Part model, mm, in its own coordinate system. A direction names the side the tool comes from. Give positions to 0.01 mm unless a question says otherwise; leave off trailing zeros. Order: outer loops, then holes, each group sorted by start corner. A loop starts at its lowest first (then second) coordinate and runs counter-clockwise, first axis right, second up. Notation, with made-up numbers: M 19,-4.5 L 45,-4.5 A14 cw 45,3.5 Z; hole C -27,33.5 d7. An arc over 180 degrees is marked long. Answer as a JSON object with one key per item and string values.
from build123d import *

# Parameters (mm, degrees)
F1_DEPTH    = 8
F2_T1_DEPTH = 8


# Not quite as in the source:
# - a fillet or chamfer that OpenCascade refuses, or shapes differently, is made with other operations: its cross-section is extruded or revolved along the edge and cut away or added


with BuildPart() as f1:
    # F0 (on Top) → F1 (new body)
    with BuildSketch(Plane.XY):
        with BuildLine():
            ThreePointArc((12.9113873807, 7.6351866975), (14.4684278813, 3.9578522768), (15, 0))
            ThreePointArc((15, 0), (14.4684278813, -3.9578522768), (12.9113873807, -7.6351866975))
            Line((12.9113873807, -7.6351866975), (18.4852353, -7.6351866975))
            ThreePointArc((18.4852353, -7.6351866975), (19.6176541156, -3.8919978161), (20, 0))
            ThreePointArc((20, 0), (19.6176541156, 3.8919978161), (18.4852353, 7.6351866975))
            Line((18.4852353, 7.6351866975), (12.9113873807, 7.6351866975))
        make_face()
        with BuildLine():
            ThreePointArc((-12.9113873807, 7.6351866975), (0, 15), (12.9113873807, 7.6351866975))
            Line((12.9113873807, 7.6351866975), (18.4852353, 7.6351866975))
            ThreePointArc((18.4852353, 7.6351866975), (0, 20), (-18.4852353, 7.6351866975))
            Line((-18.4852353, 7.6351866975), (-12.9113873807, 7.6351866975))
        make_face()
        with BuildLine():
            Line((18.4852353, -7.6351866975), (12.9113873807, -7.6351866975))
            ThreePointArc((12.9113873807, -7.6351866975), (0, -15), (-12.9113873807, -7.6351866975))
            Line((-12.9113873807, -7.6351866975), (-18.4852353, -7.6351866975))
            ThreePointArc((-18.4852353, -7.6351866975), (0, -20), (18.4852353, -7.6351866975))
        make_face()
        with BuildLine():
            ThreePointArc((-12.9113873807, -7.6351866975), (-15, 0), (-12.9113873807, 7.6351866975))
            Line((-12.9113873807, 7.6351866975), (-18.4852353, 7.6351866975))
            ThreePointArc((-18.4852353, 7.6351866975), (-20, 0), (-18.4852353, -7.6351866975))
            Line((-18.4852353, -7.6351866975), (-12.9113873807, -7.6351866975))
        make_face()
        with BuildLine():
            Line((21.6526307541, 7.6351866975), (18.4852353, 7.6351866975))
            ThreePointArc((18.4852353, 7.6351866975), (19.6176541156, 3.8919978161), (20, 0))
            ThreePointArc((20, 0), (19.6176541156, -3.8919978161), (18.4852353, -7.6351866975))
            Line((18.4852353, -7.6351866975), (21.6526307541, -7.6351866975))
            ThreePointArc((21.6526307541, -7.6351866975), (20.1620412737, 0), (21.6526307541, 7.6351866975))
        make_face()
        with BuildLine():
            ThreePointArc((-18.4852353, -7.6351866975), (-20, 0), (-18.4852353, 7.6351866975))
            Line((-18.4852353, 7.6351866975), (-21.5730507637, 7.6351866975))
            ThreePointArc((-21.5730507637, 7.6351866975), (-20.4496870957, 3.8908164426), (-20.0704748243, 0))
            ThreePointArc((-20.0704748243, 0), (-20.4496870957, -3.8908164426), (-21.5730507637, -7.6351866975))
            Line((-21.5730507637, -7.6351866975), (-18.4852353, -7.6351866975))
        make_face()
        with BuildLine():
            Line((27.135123316, 7.6351866975), (21.6526307541, 7.6351866975))
            ThreePointArc((21.6526307541, 7.6351866975), (20.1620412737, 0), (21.6526307541, -7.6351866975))
            Line((21.6526307541, -7.6351866975), (27.135123316, -7.6351866975))
            Line((27.135123316, -7.6351866975), (27.135123316, -7.5155344287))
            ThreePointArc((27.135123316, -7.5155344287), (25.1620412737, 0), (27.135123316, 7.5155344287))
            Line((27.135123316, 7.5155344287), (27.135123316, 7.6351866975))
        make_face()
        with BuildLine():
            ThreePointArc((60.7620412737, 0), (44.3517049129, 19.9238680174), (21.6526307541, 7.6351866975))
            Line((21.6526307541, 7.6351866975), (27.135123316, 7.6351866975))
            Line((27.135123316, 7.6351866975), (27.135123316, 7.5155344287))
            ThreePointArc((27.135123316, 7.5155344287), (44.347151005, 14.7985108162), (55.7620412737, 0))
            ThreePointArc((55.7620412737, 0), (44.347151005, -14.7985108162), (27.135123316, -7.5155344287))
            Line((27.135123316, -7.5155344287), (27.135123316, -7.6351866975))
            Line((27.135123316, -7.6351866975), (21.6526307541, -7.6351866975))
            ThreePointArc((21.6526307541, -7.6351866975), (44.3517049129, -19.9238680174), (60.7620412737, 0))
        make_face()
        with BuildLine():
            Line((-27.135123316, 7.6351866975), (-21.5730507637, 7.6351866975))
            ThreePointArc((-21.5730507637, 7.6351866975), (-60.3704748243, 0), (-21.5730507637, -7.6351866975))
            Line((-21.5730507637, -7.6351866975), (-27.135123316, -7.6351866975))
            ThreePointArc((-27.135123316, -7.6351866975), (-55.3704748243, 0), (-27.135123316, 7.6351866975))
        make_face()
        with BuildLine():
            ThreePointArc((-20.0704748243, 0), (-20.4496870957, 3.8908164426), (-21.5730507637, 7.6351866975))
            Line((-21.5730507637, 7.6351866975), (-27.135123316, 7.6351866975))
            ThreePointArc((-27.135123316, 7.6351866975), (-25.5957427695, 3.9547076156), (-25.0704748243, 0))
            ThreePointArc((-25.0704748243, 0), (-25.5957427695, -3.9547076156), (-27.135123316, -7.6351866975))
            Line((-27.135123316, -7.6351866975), (-21.5730507637, -7.6351866975))
            ThreePointArc((-21.5730507637, -7.6351866975), (-20.4496870957, -3.8908164426), (-20.0704748243, 0))
        make_face()
    extrude(amount=F1_DEPTH)

    # F2: chamfer of 1 on 13 edges, made by hand

    # F2_s2 → F2_t1 (join)
    with BuildSketch(Plane.XY):
        with BuildLine():
            Line((20.9909460118, -7.6351866975), (21.9050819396, -8.2297788713))
            ThreePointArc((21.9050819396, -8.2297788713), (21.7829852925, -7.9487651651), (21.6526307541, -7.6351866975))
            Line((21.6526307541, -7.6351866975), (20.9909460118, -7.6351866975))
        make_face()
        with BuildLine():
            Line((-19.1424541452, -7.6351866975), (-18.2309087097, -8.2239873309))
            ThreePointArc((-18.2309087097, -8.2239873309), (-18.3538297184, -7.9458753243), (-18.4852353, -7.6351866975))
            Line((-18.4852353, -7.6351866975), (-19.1424541452, -7.6351866975))
        make_face()
        with BuildLine():
            Line((21.9050819396, 8.2297788713), (20.9909460118, 7.6351866975))
            Line((20.9909460118, 7.6351866975), (21.6526307541, 7.6351866975))
            ThreePointArc((21.6526307541, 7.6351866975), (21.7829852925, 7.9487651651), (21.9050819396, 8.2297788713))
        make_face()
        with BuildLine():
            Line((-18.2309087097, 8.2239873309), (-19.1424541452, 7.6351866975))
            Line((-19.1424541452, 7.6351866975), (-18.4852353, 7.6351866975))
            ThreePointArc((-18.4852353, 7.6351866975), (-18.3538297184, 7.9458753243), (-18.2309087097, 8.2239873309))
        make_face()
        with BuildLine():
            Line((19.1424541452, 7.6351866975), (18.2309087097, 8.2239873309))
            ThreePointArc((18.2309087097, 8.2239873309), (18.3538297184, 7.9458753243), (18.4852353, 7.6351866975))
            Line((18.4852353, 7.6351866975), (19.1424541452, 7.6351866975))
        make_face()
        with BuildLine():
            Line((19.1424541452, -7.6351866975), (18.2309087097, -8.2239873309))
            ThreePointArc((18.2309087097, -8.2239873309), (18.3538297184, -7.9458753243), (18.4852353, -7.6351866975))
            Line((18.4852353, -7.6351866975), (19.1424541452, -7.6351866975))
        make_face()
        with BuildLine():
            Line((-21.8264389289, -8.2269036385), (-20.9135835494, -7.6351866975))
            Line((-20.9135835494, -7.6351866975), (-21.5730507637, -7.6351866975))
            ThreePointArc((-21.5730507637, -7.6351866975), (-21.703929906, -7.9473306392), (-21.8264389289, -8.2269036385))
        make_face()
    extrude(amount=F2_T1_DEPTH)

    # F2_s3 → F2_t4 (revolve, cut)
    with BuildSketch(Plane(origin=(-10.2155381424, -17.5076147757, 0), x_dir=(0, 0, 1), z_dir=(0.5039727193, 0.8637195715, 0))):
        Polygon((8, -18.5892112809), (7, -19.5892112809), (8, -19.5892112809), align=None)
    revolve(axis=Axis((-40.2204748243, 0, 8), (0, 0, -1)), mode=Mode.SUBTRACT)

    # F2_s5 → F2_t6 (revolve, cut)
    with BuildSketch(Plane(origin=(0, 0, 0), x_dir=(0, 0, 1), z_dir=(0.5090124465, -0.8607591587, 0))):
        Polygon((7, 15), (8, 16), (8, 15), align=None)
    revolve(axis=Axis((0, 0, 8), (0, 0, -1)), mode=Mode.SUBTRACT)

    # F2_s7 → F2_t8 (revolve, cut)
    with BuildSketch(Plane(origin=(9.7630309126, 17.3122900606, 0), x_dir=(0, 0, 1), z_dir=(-0.4912114006, -0.8710403894, 0))):
        Polygon((8, -18.9440721866), (7, -19.9440721866), (8, -19.9440721866), align=None)
    revolve(axis=Axis((40.4620412737, 0, 8), (0, 0, -1)), mode=Mode.SUBTRACT)

    # F2_s9 → F2_t10 (revolve, cut)
    with BuildSketch(Plane(origin=(-10.2155381424, -17.5076147757, 0), x_dir=(0, 0, 1), z_dir=(0.5039727193, 0.8637195715, 0))):
        Polygon((0, -18.5892112809), (1, -19.5892112809), (0, -19.5892112809), align=None)
    revolve(axis=Axis((-40.2204748243, 0, 0), (0, 0, -1)), mode=Mode.SUBTRACT)

    # F2_s11 → F2_t12 (revolve, cut)
    with BuildSketch(Plane(origin=(0, 0, 0), x_dir=(0, 0, 1), z_dir=(0.5090124465, -0.8607591587, 0))):
        Polygon((1, 15), (0, 16), (0, 15), align=None)
    revolve(axis=Axis((0, 0, 0), (0, 0, -1)), mode=Mode.SUBTRACT)

    # F2_s13 → F2_t14 (revolve, cut)
    with BuildSketch(Plane(origin=(9.7630309126, 17.3122900606, 0), x_dir=(0, 0, 1), z_dir=(-0.4912114006, -0.8710403894, 0))):
        Polygon((0, -18.9440721866), (1, -19.9440721866), (0, -19.9440721866), align=None)
    revolve(axis=Axis((40.4620412737, 0, 0), (0, 0, -1)), mode=Mode.SUBTRACT)


solid = f1.part
1. Probe line 1 along Y through (x, z) = (40, 1.5); line 2 along X through (y, z) = (-7, 7.75); line 3 along X through (y, z) = (12, 2.75). List the from-to ranges inside material, lowest first.
Worked answers:
{"line 1": "y = -20.29 to -15.29, 15.29 to 20.29", "line 2": "x = -59.12 to -54.5, -25.94 to -14.11, 14.11 to 26.02, 54.91 to 59.52", "line 3": "x = -56.41 to -49.47, -30.97 to -24.03, -16 to -9, 9 to 16, 24.09 to 30.97, 49.95 to 56.84"}
2. Which spindle directions (+Z, -Z, +X, -X, +Y, -Y) get a long thin tool onto all of the face, cutting with end or side? Do faces 1 (the flat face through (-0.1, -16.4, 8)), 2 (the flat face through (-20, 7.635, 4)). Say none if no direction does.
Worked answers:
{"face 1": "+Z, +X, -X, +Y, -Y", "face 2": "+Z, -Z, +Y"}
3. Cut at B-B on y = 10. State how many separate pieces and enclosed holes the cut face has, plus the area to 3 significant figures.
Worked answers:
{"separate pieces": "6", "enclosed holes": "0", "area": "286 mm^2"}
4. Pin check, flat tips, straight feed: P1, Ø1.5, axis at y = -9.5, z = 3.5, coming from the +X side; P2, Ø1.9, axis at x = -20.5, z = 4, coming from the -Y side; P3, Ø5, axis at x = 42.5, y = -13.5, coming from the +Z side. Stop position of each tip, or through.
Worked answers:
{"P1": "stops at x = 58.78", "P2": "stops at y = -7.98", "P3": "stops at z = 7.85"}
5. Cut at A-A on x = 0. Give the cut face in (y, z), plus the area to 3 significant figures.
Worked answers:
{"outline": "M -20,0 L -16,0 L -15,1 L -15,7 L -16,8 L -20,8 Z; M 15,1 L 16,0 L 20,0 L 20,8 L 16,8 L 15,7 Z", "area": "78.0 mm^2"}
